```python
from build123d import *

# Parameters (mm, degrees)
F0_W     = 78.4944
F0_H     = 80.146916
F1_DEPTH = 25.4
F2_R     = 14.863696
F3_DEPTH = 25.4
F5_DEPTH = 21.336


with BuildPart() as f1:
    # F0 (on Top) → F1 (new body)
    with BuildSketch(Plane.XY):
        Rectangle(F0_W, F0_H)
    extrude(amount=F1_DEPTH)

    # F2 (on face) → F3 (join)
    with BuildSketch(Plane.XY.offset(25.4)):
        Circle(F2_R)
    extrude(amount=F3_DEPTH)

    # F4 (on Front) → F5 (cut, symmetric)
    with BuildSketch(Plane.XZ):
        Polygon((26.566675, 57.633717), (-36.728796, 57.633717), (26.566675, 33.534981), align=None)
    extrude(amount=F5_DEPTH, both=True, mode=Mode.SUBTRACT)


solid = f1.part
```
Here's how the part is built. I have some questions about the finished solid (model axes, mm). A direction names the side the tool comes from. Coordinates: 2 decimals unless noted, no trailing zeros. Order: outer loops, then holes, each group sorted by start corner. A loop starts at its lowest first (then second) coordinate and runs counter-clockwise, first axis right, second up. Notation, with made-up numbers: (78, 7) - (107, 7) arc R20 cw to (107, 39) - close; hole circle Ø6 at (-13, 9). An arc over 180 degrees is marked (long way). One line per question, with ' | ' between items. Start each with the question number.
1. I'm going to push a flat-ended pin straight in: pin 1 Ø23.5 at (x, y) = (-1, -4.5) entering from +Z. Where does the tip first touch, or does it pass through?
2. If we section it at C-C (x = 33.5): Write out the boundary of the cut face in (y, z).
3. If we section it at B-B (x = 0): Write out the boundary of the cut face in (y, z), and give its area (3 significant figures).
4. If we section it at D-D (y = 30.5): Write out the boundary of the cut face in (x, z).
5. If we section it at A-A (y = 0): Write out the boundary of the cut face in (x, z), and give its area (3 significant figures).
6. Which directions (+Z, -Z, +X, -X, +Y, -Y) give clear straight access to the entire face, cutting with the end or side of a thin tool? Please do faces 1 (the flat face through (-1, 1, 0)), 2 (the flat face through (17, 1, 25.4)).
7. Please list where these lines run through material, in increasing order: line 1 along Z through (x, y) = (-26.5, -6); line 2 along Z through (x, y) = (11.5, -4); line 3 along Y through (x, z) = (0, 37). Write a range as [from, to].
Model answer:
1) pin 1: stops at z = 48.5
2) outline: (-40.07, 0) - (40.07, 0) - (40.07, 25.4) - (-40.07, 25.4) - close
3) outline: (-40.07, 0) - (40.07, 0) - (40.07, 25.4) - (14.86, 25.4) - (14.86, 43.65) - (-14.86, 43.65) - (-14.86, 25.4) - (-40.07, 25.4) - close | area: 2,580 mm²
4) outline: (-39.25, 0) - (39.25, 0) - (39.25, 25.4) - (-39.25, 25.4) - close
5) outline: (-39.25, 0) - (39.25, 0) - (39.25, 25.4) - (14.86, 25.4) - (14.86, 37.99) - (-14.86, 49.31) - (-14.86, 25.4) - (-39.25, 25.4) - close | area: 2,540 mm²
6) face 1: -Z, +X, -X, +Y, -Y | face 2: +Z
7) line 1: z = [0, 25.4] | line 2: z = [0, 39.27] | line 3: y = [-14.86, 14.86]
